Verification items for this drawing (mm, ordinates from the low corner). A direction names the side the tool comes from. Give positions to 0.01 mm unless a question says otherwise; leave off trailing zeros. Write each loop counter-clockwise with the first axis right and the second up, starting at its lowest first coordinate (ties: lowest second). Pieces come first, ordered by that corner, then holes. Notation, with made-up numbers: (39.25, 37.25) -> (87.25, 37.25) arc R29 cw to (87.25, 69.25) -> close; hole circle Ø1 at (-16, 22). An arc over 180 degrees is marked (long way). Use one line per item in the form item = value. Start each with the question number.
(1) Scan lines: L1, parallel to Y at x = 7, z = 3.75; L2, parallel to Y at x = 10.5, z = 0.75; L3, parallel to Y at x = 7.75, z = 2.3. Record each from-to range of solid material in increasing order.
(2) Set-up check for the marked faces 4 and 5: record each of +Z, -Z, +X, -X, +Y, -Y from which the full face is reachable in a straight line by a thin tool's end or side.
(3) Section check D-D, the plane y = 38. Record the cut outline in (x, z), plus the area to 3 significant figures.
(4) Section check A-A, the plane x = 7. Record the cut outline in (y, z), plus the area to 3 significant figures.
(5) Section check C-C, the plane z = 0.95. Record the cut outline in (x, y).
(6) Section check B-B, the plane y = 7. Record the cut outline in (x, z).
(7) Release check for a two-part mould opening along X. For the marked faces 1, 2 and 3 record: pulls with the +X half, pulls with the -X half, needs draft (parallel to the pull), parting line crosses it, or undercut.
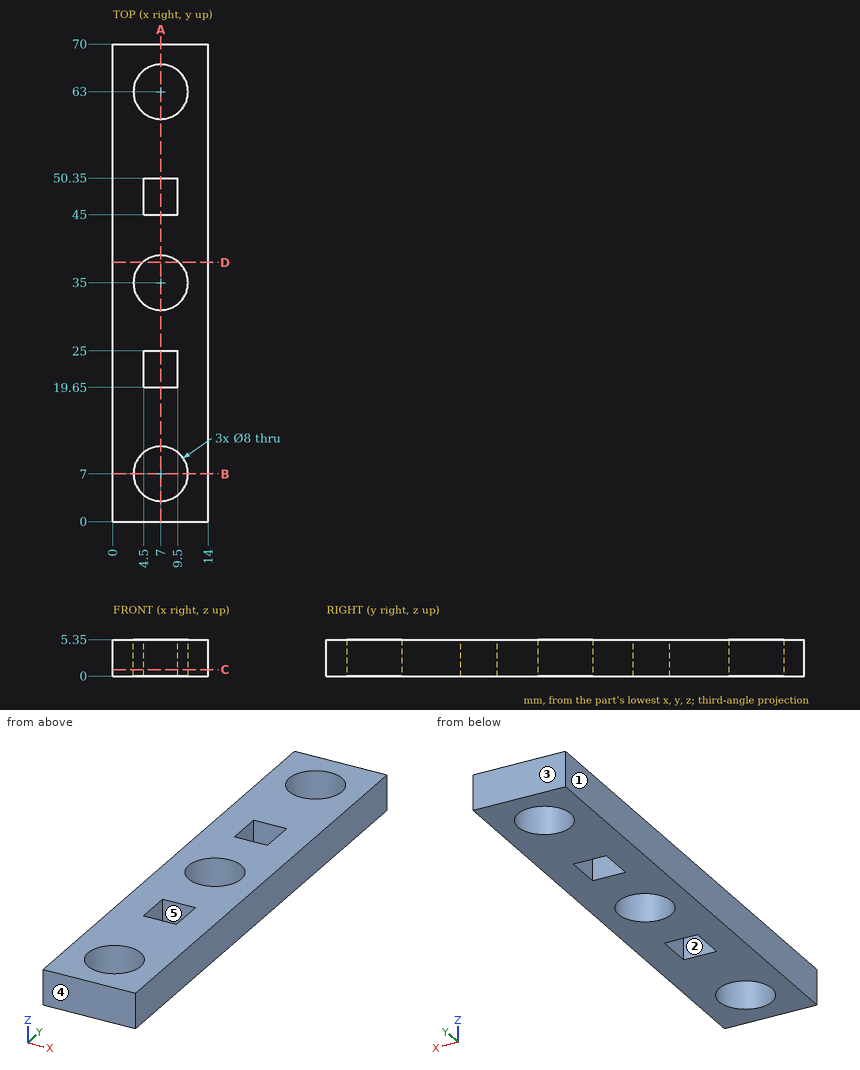
Completed:
q1.L1 = 0 to 3, 11 to 19.65, 25 to 31, 39 to 45, 50.35 to 59, 67 to 70
q1.L2 = 0 to 5.06, 8.94 to 33.06, 36.94 to 61.06, 64.94 to 70
q1.L3 = 0 to 3.07, 10.93 to 19.65, 25 to 31.07, 38.93 to 45, 50.35 to 59.07, 66.93 to 70
q2.face_4 = +Z, -Z, +X, -X, -Y
q2.face_5 = +Z, -Z
q3.outline = (0, 0) -> (4.35, 0) -> (4.35, 5.35) -> (0, 5.35) -> close; (9.65, 0) -> (14, 0) -> (14, 5.35) -> (9.65, 5.35) -> close
q3.area = 46.6 mm²
q4.outline = (0, 0) -> (3, 0) -> (3, 5.35) -> (0, 5.35) -> close; (11, 0) -> (19.65, 0) -> (19.65, 5.35) -> (11, 5.35) -> close; (25, 0) -> (31, 0) -> (31, 5.35) -> (25, 5.35) -> close; (39, 0) -> (45, 0) -> (45, 5.35) -> (39, 5.35) -> close; (50.35, 0) -> (59, 0) -> (59, 5.35) -> (50.35, 5.35) -> close; (67, 0) -> (70, 0) -> (70, 5.35) -> (67, 5.35) -> close
q4.area = 189 mm²
q5.outline = (0, 0) -> (14, 0) -> (14, 70) -> (0, 70) -> close; hole circle Ø8 at (7, 7); hole circle Ø8 at (7, 35); hole circle Ø8 at (7, 63); hole (4.5, 19.65) -> (9.5, 19.65) -> (9.5, 25) -> (4.5, 25) -> close; hole (4.5, 45) -> (9.5, 45) -> (9.5, 50.35) -> (4.5, 50.35) -> close
q6.outline = (0, 0) -> (3, 0) -> (3, 5.35) -> (0, 5.35) -> close; (11, 0) -> (14, 0) -> (14, 5.35) -> (11, 5.35) -> close
q7.face_1 = pulls with the -X half
q7.face_2 = undercut
q7.face_3 = needs draft
